Autodesk Inventor part; units mm, degrees
ref_plane "YZ Plane" through (0, 0, 0) normal (1, 0, 0) x (0, 1, 0)
ref_plane "XZ Plane" through (0, 0, 0) normal (0, 1, 0) x (-1, 0, 0)
ref_plane "XY Plane" through (0, 0, 0) normal (0, 0, 1) x (1, 0, 0)
sketch "Boceto1" plane through (0, 0, 0) normal (0, 0, 1) x (1, 0, 0)
  circle A0 centre (0, 0) radius 20
  circle A1 centre (0, 0) radius 4
  dimension "d0" = 40
  dimension "d42" = 8
extrude "Extrusión1" add sketch "Boceto1" along normal blind 5
sketch "Boceto3" plane through (0, 0, 0) normal (0, 0, -1) x (-1, 0, 0)
  circle A0 centre (0, 15) radius 2
  circle A1 centre (-15, 0) radius 2
  circle A2 centre (15, 0) radius 2
  circle A3 centre (0, -15) radius 2
  point P0 (0, 0)
  dimension "d6" = 4
  dimension "d7" = 4
  dimension "d8" = 4
  dimension "d9" = 4
  dimension "d10" = 15
  dimension "d11" = 15
  dimension "d12" = 15
  dimension "d13" = 15
hole "Agujero1" at (0, 15, 0) direction (0, 0, 1) diameter 4 end through all
hole "Agujero2" at (15, 0, 0) direction (0, 0, 1) diameter 4 end through all
hole "Agujero3" at (-15, 0, 0) direction (0, 0, 1) diameter 4 end through all
hole "Agujero4" at (0, -15, 0) direction (0, 0, 1) diameter 4 end through all
properties part number "Brida1"
Could you check a few things on this model? Use its own coordinates, in mm. Give positions to 0.01 mm unless a question says otherwise; leave off trailing zeros. Loops run counter-clockwise (first coordinate to the right, second up) from the corner with the lowest first, then second, coordinate; pieces in that order, holes last. Notation, with made-up numbers: (36.5, 13) - (50.5, 13) arc R24 cw to (50.5, 45) - close; hole circle Ø11 at (54, 8). An arc over 180 degrees is marked (long way). Use one line per item in the form item = value.
1. I want a section at A-A (x = 0). Please give me the cut outline in (y, z).
Response values:
outline = (-20, 0) - (-17, 0) - (-17, 5) - (-20, 5) - close; (-13, 0) - (-4, 0) - (-4, 5) - (-13, 5) - close; (4, 0) - (13, 0) - (13, 5) - (4, 5) - close; (17, 0) - (20, 0) - (20, 5) - (17, 5) - close
2. I want a section at C-C (x = -15.5). Please give me the cut outline in (y, z).
Response values:
outline = (-12.64, 0) - (-1.94, 0) - (-1.94, 5) - (-12.64, 5) - close; (1.94, 0) - (12.64, 0) - (12.64, 5) - (1.94, 5) - close
3. I want a section at B-B (y = 14.5). Please give me the cut outline in (x, z).
Response values:
outline = (-13.77, 0) - (-1.94, 0) - (-1.94, 5) - (-13.77, 5) - close; (1.94, 0) - (13.77, 0) - (13.77, 5) - (1.94, 5) - close
4. I'm going to push flat-ended pins straight in: pin 1 Ø10 at (x, y) = (-11.5, -9) entering from -Z; pin 2 Ø2 at (x, z) = (-11.5, 2) entering from +Y; pin 3 Ø1.5 at (x, z) = (14, 4) entering from +Y; pin 4 Ø1 at (y, z) = (14, 2) entering from -X. Where does each tip first touch, or does it pass through?
Response values:
pin_1 = 0
pin_2 = 17.02
pin_3 = 14.98
pin_4 = -14.76
5. I need wall thicknesses on probe 1 along Y at (x, z) = (0, 2.8); probe 2 along X at (y, z) = (-0.5, 2.35); probe 3 along Y at (x, z) = (16.5, 4.05). Which ranges of each line are inside material? Lowest first, please.
Response values:
probe_1 = -20 to -17, -13 to -4, 4 to 13, 17 to 20
probe_2 = -19.99 to -16.94, -13.06 to -3.97, 3.97 to 13.06, 16.94 to 19.99
probe_3 = -11.3 to -1.32, 1.32 to 11.3
6. Thinking about a two-plate mould opening in X: for faces 1 (the face through (-4.336, 19.524, 2.465)), 2 (the face through (13, 0, 3)), 3 (the face through (4.2, 0.3, 0)), which applies, released by +X, released by -X, zero draft, split by the parting line, or undercut?
Response values:
face_1 = split by the parting line
face_2 = undercut
face_3 = zero draft
